from build123d import *

# Parameters (mm, degrees)
ESQUISSE1_R             = 14
BOSS_EXTRU_1_DEPTH      = 2.2
ESQUISSE2_R             = 12.8
BOSS_EXTRU_2_DEPTH      = 1.4
ESQUISSE3_R             = 8
BOSS_EXTRU_3_DEPTH      = 1.7
ESQUISSE4_R             = 12.5
ENL_V_MAT_EXTRU_1_DEPTH = 1
CONG_1_R                = 0.6


with BuildPart() as part:
    # Esquisse1 → Boss.-Extru.1 (new body)
    with BuildSketch(Plane.XY):
        Circle(ESQUISSE1_R)
    extrude(amount=BOSS_EXTRU_1_DEPTH)

    # Esquisse2 → Boss.-Extru.2 (add)
    with BuildSketch(Plane.XY.offset(2.2)):
        Circle(ESQUISSE2_R)
    extrude(amount=BOSS_EXTRU_2_DEPTH)

    # Esquisse3 → Boss.-Extru.3 (add)
    with BuildSketch(Plane.XY.offset(3.6)):
        Circle(ESQUISSE3_R)
    extrude(amount=BOSS_EXTRU_3_DEPTH)

    # Esquisse4 → Enlèv. mat.-Extru.1 (cut)
    with BuildSketch(Plane(origin=(0, 0, 0), x_dir=(-1, 0, 0), z_dir=(0, 0, -1))):
        Circle(ESQUISSE4_R)
    extrude(amount=-ENL_V_MAT_EXTRU_1_DEPTH, mode=Mode.SUBTRACT)

    # Congé1
    cong_1_edges = [part.edges().sort_by_distance(p)[0] for p in [
        (-8, 0, 5.3),
        (-14, 0, 2.2),
        (-12.8, 0, 3.6),
    ]]
    fillet(cong_1_edges, radius=CONG_1_R)


solid = part.part
Geometry: final body of the model. Coordinates: model frame, mm. A direction names the side the tool comes from. Give positions to 0.01 mm unless a question says otherwise; leave off trailing zeros. Loops run counter-clockwise (first coordinate to the right, second up) from the corner with the lowest first, then second, coordinate; pieces in that order, holes last. Notation, with made-up numbers: M -21,-17.75 L 35,-17.75 A21 ccw 35,3.25 Z; hole C 53,13.5 d2. An arc over 180 degrees is marked long. Put each result on its own line as item: value. Start each with the question number.
1) Cut plane A-A (y = 0). Output: boundary loops of the cut face in (x, z), then the cut area to 3 significant figures.
2) Access query for faces 1 (the cylindrical face through (-10.158, -7.789, 2.594)), 2 (the cylindrical face through (12.932, -5.362, 0.789)), 3 (the cylindrical face through (-11.923, 3.755, 0.493)). Directions: +Z, -Z, +X, -X, +Y, -Y. A direction counts if a zero-diameter tool reaches every point of the face in a straight line with its end or side. Return the directions, or none.
3) Contact query for flat-ended pins moving along their axis: pin 1 (1 mm diameter, centred on x = -2.5, y = -1, fed in from -Z); pin 2 (3 mm diameter, centred on x = -7.5, z = 3.5, fed in from +Y); pin 3 (1 mm diameter, centred on x = -11, z = 2.5, fed in from +Y). Output: stop coordinate, or through.
4) Pull-direction query (X, two-part tool) for faces 4 (the flat face through (7, -11, 2.2)), 5 (the flat face through (0, 0, 1)), 6 (the cylindrical face through (-1.73, -7.81, 4.14)); classes: pulls with the +X half, pulls with the -X half, needs draft (parallel to the pull), parting line crosses it, or undercut.
5) Cut plane D-D (z = 4.1). Output: boundary loops of the cut face in (x, y), then the cut area to 3 significant figures.
6) Cut plane C-C (z = 2.65). Output: boundary loops of the cut face in (x, y).
7) Ray query, line 1 along Y through (x, z) = (0, 0.65); line 2 along Z through (x, y) = (-5.5, -1.75); line 3 along Z through (x, y) = (-11.5, -3.5). Return the intervals inside material, ascending.
Verdict:
1. outline: M -14,0 L -12.5,0 L -12.5,1 L 12.5,1 L 12.5,0 L 14,0 L 14,1.6 A0.6 ccw 13.4,2.2 L 12.8,2.2 L 12.8,3 A0.6 ccw 12.2,3.6 L 8,3.6 L 8,4.7 A0.6 ccw 7.4,5.3 L -7.4,5.3 A0.6 ccw -8,4.7 L -8,3.6 L -12.2,3.6 A0.6 ccw -12.8,3 L -12.8,2.2 L -13.4,2.2 A0.6 ccw -14,1.6 Z
1. area: 99.2 mm2
2. face 1: +Z
2. face 2: +Z, -Z
2. face 3: -Z
3. pin 1: z = 1
3. pin 2: y = 11.84
3. pin 3: y = 8.62
4. face 4: needs draft
4. face 5: undercut
4. face 6: parting line crosses it
5. outline: C 0,0 d16
5. area: 201 mm2
6. outline: C 0,0 d25.6
7. line 1: -14 to -12.5, 12.5 to 14
7. line 2: 1 to 5.3
7. line 3: 1 to 3.6
